Source: CAD feature listing. Evaluate the final solid. Frame: model axes, mm. A direction names the side the tool comes from. Give positions to 0.01 mm unless a question says otherwise; leave off trailing zeros. Order: outer loops, then holes, each group sorted by start corner. A loop starts at its lowest first (then second) coordinate and runs counter-clockwise, first axis right, second up. Notation, with made-up numbers: (43, 22) - (75, 22) arc R32 ccw to (75, 59) - close; hole circle Ø6 at (19.5, 66). An arc over 180 degrees is marked (long way). One line per item, written item: value. Start each with the question number.
Autodesk Inventor part; units mm, degrees
ref_plane "Work Plane1" through (0, 0, 0) normal (0, 0, 1) x (1, 0, 0)
ref_plane "YZ Plane" through (0, 0, 0) normal (1, 0, 0) x (0, 1, 0)
ref_plane "XZ Plane" through (0, 0, 0) normal (0, 1, 0) x (-1, 0, 0)
sketch "Sketch2" plane through (0, 0, 0) normal (0, 0, 1) x (1, 0, 0)
  circle A0 centre (0, 277.5) radius 8 construction
  circle A1 centre (0, 277.5) radius 13
  circle A2 centre (0, 277.5) radius 10.5 construction
  line L0 (25, 287.5) -> (-25, 287.5) construction
  line L1 (-25, 287.5) -> (-25, 222.5) construction
  line L2 (-25, 222.5) -> (25, 222.5) construction
  line L3 (25, 222.5) -> (25, 287.5) construction
  circle A3 centre (15, 228.5) radius 2.7
  circle A4 centre (-15, 228.5) radius 2.7
  circle A5 centre (-19, 277.5) radius 2.7
  circle A6 centre (19, 277.5) radius 2.7
  circle A7 centre (0, -277.5) radius 8 construction
  circle A8 centre (0, -277.5) radius 13
  circle A9 centre (0, -277.5) radius 10.5 construction
  line L4 (25, -287.5) -> (-25, -287.5) construction
  line L5 (-25, -287.5) -> (-25, -222.5) construction
  line L6 (-25, -222.5) -> (25, -222.5) construction
  line L7 (25, -222.5) -> (25, -287.5) construction
  circle A10 centre (-15, -228.5) radius 2.7
  circle A11 centre (15, -228.5) radius 2.7
  circle A12 centre (-19, -277.5) radius 2.7
  circle A13 centre (19, -277.5) radius 2.7
  line L8 (10.5, -277.5) -> (10.5, -287.5) construction
  line L9 (-10.5, -277.5) -> (-10.5, -287.5) construction
  line L10 (10.5, 277.5) -> (10.5, 287.5) construction
  line L11 (-10.5, 277.5) -> (-10.5, 287.5) construction
  circle A14 centre (281.7, 0) radius 5.25
  circle A15 centre (-281.7, 0) radius 5.25
  line L12 (0, -321.7336) -> (321.7336, 0)
  line L13 (321.7336, 0) -> (0, 321.7336)
  line L14 (0, 321.7336) -> (-321.7336, 0)
  line L15 (-321.7336, 0) -> (0, -321.7336)
  line L16 (321.7336, 0) -> (-321.7336, 0) construction
  line L17 (0, -321.7336) -> (455, -321.7336) construction
  line L18 (300.5, 21.2336) -> (300.5, -21.2336)
  line L19 (-300.5, 21.2336) -> (-300.5, -21.2336)
  line L20 (-24.2336, 297.5) -> (24.2336, 297.5) construction
  line L21 (-29.2336, 292.5) -> (29.2336, 292.5)
  line L22 (-24.2336, -297.5) -> (24.2336, -297.5) construction
  line L23 (-29.2336, -292.5) -> (29.2336, -292.5)
  line L24 (-9.5, 297.5) -> (-3.976, 284.442) construction
  line L25 (9.5, 297.5) -> (3.976, 284.442) construction
  line L26 (-14.929, 297.5) -> (-9.9883, 285.8207)
  line L27 (14.929, 297.5) -> (9.9883, 285.8207)
  line L28 (-9.5, -297.5) -> (-3.976, -284.442) construction
  line L29 (9.5, -297.5) -> (3.976, -284.442) construction
  line L30 (14.929, -297.5) -> (9.9883, -285.8207)
  line L31 (-14.929, -297.5) -> (-9.9883, -285.8207)
  line L32 (13, 277.5) -> (13, 292.5)
  line L33 (-13, 277.5) -> (-13, 292.5)
  line L34 (-13, -277.5) -> (-13, -292.5)
  line L35 (13, -277.5) -> (13, -292.5)
  line L36 (281.7, 0) -> (287.3569, 5.6569) construction
  line L37 (281.7, 0) -> (289.7, 0) construction
  circle A16 centre (287.3569, 5.6569) radius 1.6
  circle A17 centre (276.0431, 5.6569) radius 1.6
  circle A18 centre (276.0431, -5.6569) radius 1.6
  circle A19 centre (287.3569, -5.6569) radius 1.6
  line L38 (-281.7, 0) -> (-287.3569, 5.6569) construction
  circle A20 centre (-287.3569, 5.6569) radius 1.6
  circle A21 centre (-287.3569, -5.6569) radius 1.6
  circle A22 centre (-276.0431, -5.6569) radius 1.6
  circle A23 centre (-276.0431, 5.6569) radius 1.6
  line L39 (0, -321.7336) -> (0, 321.7336) construction
  point P0 (0, 0)
  point P1 (-12.8138, -292.5)
  point P2 (12.8138, -292.5)
  point P3 (12.8138, 292.5)
  point P4 (-12.8138, 292.5)
  point P5 (300.5, 292.5)
  point P6 (300.5, -292.5)
  point P7 (-300.5, -292.5)
  point P8 (-300.5, 292.5)
  dimension "d256" = 16
  dimension "d258" = 277.5
  dimension "d259" = 26
  dimension "d260" = 21
  dimension "d262" = 10
  dimension "d263" = 65
  dimension "d271" = 6
  dimension "d272" = 10
  dimension "d275" = 6
  dimension "d276" = 10
  dimension "d285" = 10
  dimension "d300" = 10.5
  dimension "d302" = 281.7
  dimension "d321" = 45
  dimension "d322" = 455
  dimension "d323" = 18.8
  dimension "d325" = 20
  dimension "d326" = 15
  dimension "d330" = 67.07
  dimension "d331" = 9.5
  dimension "d336" = 14.929
  dimension "d391" = 8
  dimension "d392" = 45
  dimension "d394" = 3.2
  dimension "d397" = 360
  dimension "d399" = 8
  dimension "d400" = 45
  dimension "d404" = 360
  dimension "d432" = 5.4
  dimension "d433" = 50
ref_plane "Work Plane1" through (0, 0, 0) normal (0, 0, 1) x (1, 0, 0)
sketch "Sketch3" plane through (0, 0, 0) normal (0, 0, 1) x (1, 0, 0)
  line L0 (-160.8668, -160.8668) -> (160.8668, 160.8668) construction
  line L1 (-160.8668, -160.8668) -> (294.1332, -160.8668) construction
  line L2 (279.5102, 35.1523) -> (35.1523, 279.5102) construction
  line L3 (35.1523, 279.5102) -> (6.8681, 251.2259) construction
  line L4 (6.8681, 251.2259) -> (251.2259, 6.8681) construction
  line L5 (251.2259, 6.8681) -> (279.5102, 35.1523) construction
  circle A0 centre (19, 277.5) radius 2.7
  circle A1 centre (15, 228.5) radius 2.7
  line L6 (-35.1523, -279.5102) -> (-279.5102, -35.1523) construction
  line L7 (-279.5102, -35.1523) -> (-251.2259, -6.8681) construction
  line L8 (-251.2259, -6.8681) -> (-6.8681, -251.2259) construction
  line L9 (-6.8681, -251.2259) -> (-35.1523, -279.5102) construction
  circle A2 centre (-79.5495, -185.6155) radius 3.1
  circle A3 centre (-100.7627, -206.8287) radius 3.1
  circle A4 centre (-185.6155, -79.5495) radius 3.1
  circle A5 centre (-206.8287, -100.7627) radius 3.1
  line L10 (-160.8668, 160.8668) -> (160.8668, -160.8668) construction
  circle A6 centre (206.8287, 100.7627) radius 3.1
  circle A7 centre (185.6155, 79.5495) radius 3.1
  circle A8 centre (100.7627, 206.8287) radius 3.1
  circle A9 centre (79.5495, 185.6155) radius 3.1
  line L11 (-175.0089, 138.2394) -> (-138.2394, 175.0089) construction
  line L12 (-138.2394, 175.0089) -> (-125.5115, 162.281) construction
  line L13 (-125.5115, 162.281) -> (-162.281, 125.5115) construction
  line L14 (-162.281, 125.5115) -> (-175.0089, 138.2394) construction
  circle A10 centre (-138.2394, 175.0089) radius 2.1
  circle A11 centre (-125.5115, 162.281) radius 2.1
  circle A12 centre (-162.281, 125.5115) radius 2.1
  circle A13 centre (-175.0089, 138.2394) radius 2.1
  line L15 (-162.281, 125.5115) -> (-138.2394, 175.0089) construction
  line L16 (-175.0089, 138.2394) -> (-125.5115, 162.281) construction
  line L17 (138.9465, -168.645) -> (168.645, -138.9465) construction
  circle A14 centre (168.645, -138.9465) radius 2.1
  circle A15 centre (138.9465, -168.645) radius 2.1
  line L18 (21.0102, 265.3681) -> (265.3681, 21.0102) construction
  line L19 (-265.3681, -21.0102) -> (-21.0102, -265.3681) construction
  point P0 (0, 0)
  point P1 (-150.2602, 150.2602)
  point P2 (153.7957, -153.7957)
  dimension "d349" = 455
  dimension "d350" = 45
  dimension "d353" = 40
  dimension "d354" = 10
  dimension "d362" = 75
  dimension "d363" = 5
  dimension "d365" = 5
  dimension "d366" = 75
  dimension "d370" = 5
  dimension "d371" = 75
  dimension "d373" = 5
  dimension "d374" = 75
  dimension "d436" = 52
  dimension "d437" = 18
  dimension "d438" = 221.5
  dimension "d439" = 4.2
  dimension "d440" = 42
  dimension "d442" = 217.5
  dimension "d450" = 6.2
  dimension "d482" = 405
extrude "Extrusion12" add sketch "Sketch2" against normal blind 10 contours L32 L21 L13 L18 L12 L23 L35 A8 L34 L15 L19 L14 L33 A1
hole "Hole2" at (100.7627, 206.8287, 0) at (79.5495, 185.6155, 0) at (206.8287, 100.7627, 0) at (185.6155, 79.5495, 0) at (-79.5495, -185.6155, 0) at (-100.7627, -206.8287, 0) at (-185.6155, -79.5495, 0) at (-206.8287, -100.7627, 0) direction (0, 0, -1) diameter 6.2 end through all
hole "Hole4" at (-175.0089, 138.2394, 0) at (-162.281, 125.5115, 0) at (-125.5115, 162.281, 0) at (-138.2394, 175.0089, 0) at (168.645, -138.9465, 0) at (138.9465, -168.645, 0) direction (0, 0, -1) diameter 4.2 end through all
sketch "Sketch5" plane through (0, 0, 0) normal (0, 0, 1) x (1, 0, 0)
  line L0 (29.9874, 217.5) -> (-61.8072, 217.5)
  line L1 (139.6536, -139.6536) -> (-139.6536, 139.6536) construction
  line L2 (-29.9874, -217.5) -> (-263.3973, 15.9099)
  line L3 (61.8072, -217.5) -> (-29.9874, -217.5)
  line L4 (247.4874, 0) -> (-247.4874, 0) construction
  line L5 (-61.8072, 217.5) -> (-263.3973, 15.9099)
  line L6 (61.8072, -217.5) -> (263.3973, -15.9099)
  line L7 (0, -217.5) -> (0, 217.5) construction
  line L8 (263.3973, -15.9099) -> (29.9874, 217.5)
  line L9 (-123.7437, -123.7437) -> (123.7437, 123.7437) construction
  line L10 (-217.5, 61.8072) -> (-217.5, -29.9874)
  line L11 (217.5, 29.9874) -> (217.5, -61.8072)
  line L12 (-247.4874, 0) -> (-29.9874, 217.5)
  line L13 (247.4874, 0) -> (29.9874, -217.5)
  line L14 (-7.5, 217.5) -> (-7.5, -217.5)
  line L15 (7.5, 217.5) -> (7.5, -217.5)
  line L16 (-239.9874, 7.5) -> (239.9874, 7.5)
  line L17 (239.9874, -7.5) -> (-239.9874, -7.5)
  line L18 (-239.9874, -7.5) -> (-239.9874, 39.3198)
  line L19 (239.9874, 7.5) -> (239.9874, -39.3198)
  point P0 (0, 0)
  point P1 (-7.5, -7.5)
  point P2 (7.5, -7.5)
  point P3 (-7.5, 7.5)
  point P4 (7.5, 7.5)
  point P5 (217.5, -29.9874)
  point P6 (-217.5, 29.9874)
  dimension "d460" = 197.5
  dimension "d461" = 197.5
  dimension "d465" = 175
  dimension "d466" = 217.5
  dimension "d467" = 45
  dimension "d468" = 217.5
  dimension "d469" = 175
  dimension "d473" = 15
  dimension "d475" = 15
extrude "Extrusion15" cut sketch "Sketch5" against normal blind 217.5 contours L8 L11 L16 L15 L0 | L8 L16 L11 | L14 L16 L10 L12 L0 | L12 L10 L5 L0 | L17 L11 L13 L3 L15 | L19 L6 L11 L13 | L13 L11 L17 | L12 L18 L5 L10 | L10 L16 L12 | L14 L3 L2 L10 L17 | L11 L6 L3 L13 | L10 L2 L17
fillet "Fillet2" radius 10 18 edges at (-61.8072, 217.5, -5) (29.9874, 217.5, -5) (-7.5, 217.5, -5) (239.9874, -7.5, -5) (-7.5, -7.5, -5) (239.9874, -39.3198, -5) (61.8072, -217.5, -5) (-7.5, -217.5, -5) (-7.5, 7.5, -5) (-29.9874, -217.5, -5) (7.5, 7.5, -5) (-239.9874, 7.5, -5) (-239.9874, 39.3198, -5) (7.5, -7.5, -5) (7.5, 217.5, -5) (7.5, -217.5, -5) (239.9874, 7.5, -5) (-239.9874, -7.5, -5)
equation "\"dist_rails\" = 555"
equation "\"dist_leadscrews\" = 563.4"
equation "\"diam_leadscrew_hole\" = 10.5"
equation "\"z_plate_width\" = 455"
equation "\"delta\" = 5"
equation "\"rail_angle\" = 67.07deg"
equation "\"rail_D\" = 9.5"
equation "\"rail_diam\" = 16"
equation "\"rail_dist\" = 405"
properties part number "z_plate" material "Aluminum 6061"
1. Contact query for flat-ended pins moving along their axis: pin 1 Ø6 at (x, z) = (76.5, -6) entering from +Y; pin 2 Ø3 at (y, z) = (24, -5.5) entering from +X; pin 3 Ø5 at (y, z) = (-77, -5) entering from +X. Output: stop coordinate, or through.
2. Ray query, L1, parallel to Y at x = -19, z = -5.25; L2, parallel to Y at x = 22, z = -2; L3, parallel to Y at x = 48, z = -2. Return the intervals inside material, ascending.
3. Section C-C on x = 0. Return the cut outline in (y, z).
4. Section A-A on y = -115.5. Return the cut outline in (x, z), then the cut area to 3 significant figures.
5. Section D-D on z = -6. Count the separate pieces of the cut face and the enclosed holes in it, then the cut area to 3 significant figures.
6. Section B-B on x = 120. Return the cut outline in (y, z), then the cut area to 3 significant figures.
7. Set-up query: faces 1 (the flat face through (166.766, 154.968, -4.93)), 2 (the flat face through (149.69, -129.62, -4.93)). Return all of +Z, -Z, +X, -X, +Y, -Y with unobstructed straight access to the full face (end or side cutting, diameter ignored); none if empty.
8. Draft query along X for faces 3 (the flat face through (-1, 1, 0)), 4 (the flat face through (-166.766, -154.968, -4.93)), 5 (the flat face through (-126.59, -120.9, -4.93)). Return one class per face: pulls with the +X half, pulls with the -X half, needs draft (parallel to the pull), parting line crosses it, or undercut.
Data:
1. pin 1: stops at y = 248.23
1. pin 2: stops at x = 299.23
1. pin 3: stops at x = 247.23
2. L1: y = -292.5 to -280.2, -274.8 to -217.5, -7.5 to 7.5, 217.5 to 274.8, 280.2 to 292.5
2. L2: y = -292.5 to -217.5, -7.5 to 7.5, 217.5 to 292.5
2. L3: y = -273.73 to -217.5, -7.5 to 7.5, 199.49 to 273.73
3. outline: (-264.5, -10) - (264.5, -10) - (264.5, 0) - (-264.5, 0) - close
4. outline: (-206.23, -10) - (-131.99, -10) - (-131.99, 0) - (-206.23, 0) - close; (-7.5, -10) - (7.5, -10) - (7.5, 0) - (-7.5, 0) - close; (163.81, -10) - (206.23, -10) - (206.23, 0) - (163.81, 0) - close
4. area: 1,320 mm2
5. separate pieces: 1
5. enclosed holes: 36
5. area: 83,400 mm2
6. outline: (-201.73, -10) - (-159.31, -10) - (-159.31, 0) - (-201.73, 0) - close; (-7.5, -10) - (7.5, -10) - (7.5, 0) - (-7.5, 0) - close; (127.49, -10) - (201.73, -10) - (201.73, 0) - (127.49, 0) - close
6. area: 1,320 mm2
7. face 1: +Z, -Z, +X, +Y
7. face 2: +Z, -Z
8. face 3: needs draft
8. face 4: pulls with the -X half
8. face 5: undercut
